Design review of the part built by this model. Coordinates are the model's own, in mm. Face numbers are marked on the shaded views. A direction names the side the tool comes from. Give positions to 0.01 mm unless a question says otherwise; leave off trailing zeros. Write each loop counter-clockwise with the first axis right and the second up, starting at its lowest first coordinate (ties: lowest second). Pieces come first, ordered by that corner, then holes. Notation, with made-up numbers: (-3, -9.75) -> (17, -9.75) arc R15 cw to (17, 0.25) -> close; hole circle Ø7 at (69, -18). An arc over 180 degrees is marked (long way). Use CSV: the item, a comma, the result in double quotes.
```python
from build123d import *

# Parameters (mm, degrees)
EXTRUDE_1_DEPTH     = 30
SKETCH_2_W          = 8
SKETCH_2_H          = 40
EXTRUDE_2_DEPTH     = 100
SKETCH_3_R          = 20
CUT_EXTRUDE_1_DEPTH = 211.428135001
SKETCH_5_W          = 87.00766185
SKETCH_5_H          = 105.192301749
CUT_EXTRUDE_2_DEPTH = 10


with BuildPart() as part:
    # 草图1 → 凸台-拉伸1 (new body)
    with BuildSketch(Plane(origin=(0, 0, 0), x_dir=(1, 0, 0), z_dir=(0, 1, 0))):
        with BuildLine():
            Line((-74, 20), (-71.246052522, 20))
            ThreePointArc((-71.246052522, 20), (0, 74), (71.246052522, 20))
            Line((71.246052522, 20), (74, 20))
            Line((74, 20), (74, -20))
            Line((74, -20), (66, -20))
            Line((66, -20), (66, 0))
            ThreePointArc((66, 0), (0, 66), (-66, 0))
            Line((-66, 0), (-66, -20))
            Line((-66, -20), (-74, -20))
            Line((-74, -20), (-74, 20))
        make_face()
    extrude(amount=EXTRUDE_1_DEPTH)

    # 草图2 → 凸台-拉伸2 (add)
    with BuildSketch(Plane(origin=(0, 30, 0), x_dir=(1, 0, 0), z_dir=(0, 1, 0))):
        with Locations((-70, 0)):
            Rectangle(SKETCH_2_W, SKETCH_2_H)
        with Locations((70, 0)):
            Rectangle(SKETCH_2_W, SKETCH_2_H)
    extrude(amount=EXTRUDE_2_DEPTH)

    # 草图3 → 切除-拉伸1 (cut, through all)
    with BuildSketch(Plane.ZY.offset(74)):
        with Locations((0, 146)):
            Circle(SKETCH_3_R)
    extrude(amount=-CUT_EXTRUDE_1_DEPTH, mode=Mode.SUBTRACT)

    # 草图5 → 切除-拉伸2 (cut)
    with BuildSketch(Plane(origin=(74, 0, 0), x_dir=(0, 0, -1), z_dir=(1, 0, 0))):
        with Locations((-23.503830925, 82.596150874)):
            Rectangle(SKETCH_5_W, SKETCH_5_H)
    extrude(amount=-CUT_EXTRUDE_2_DEPTH, mode=Mode.SUBTRACT)


solid = part.part
```
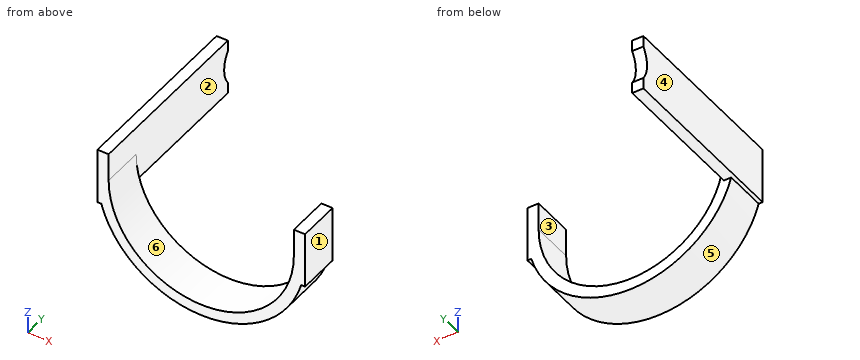
(1) For line 1 along X through (y, z) = (56, -5); line 2 along Z through (x, y) = (-19, 15); line 3 along Z through (x, y) = (-54, 29), list the stretches that pass through material, from the lowest coordinate up. Write a range as [from, to].
Established:
line 1,"x = [-74, -66]"
line 2,"z = [-71.52, -63.21]"
line 3,"z = [-50.6, -37.95]"
(2) Tool access review of the marked faces 1, 2 and 3: name each direction out of +Z, -Z, +X, -X, +Y, -Y from which nothing blocks a thin tool from reaching the whole face with its end or side.
Established:
face 1,"+Z, -Z, +X, +Y, -Y"
face 2,"+Z, +Y"
face 3,"+Z, +Y, -Y"
(3) Mouldability with a two-part tool opening along X and no side actions: class the marked faces 4, 5 and 6 as +X half, -X half, draft (parallel to the pull), parting line (faces both ways), or undercut.
Established:
face 4,"-X half"
face 5,"parting line"
face 6,"undercut"
(4) Take a section at C-C (x = 0). Write out the cut boundary in (y, z).
Established:
outline,"(0, -74) -> (30, -74) -> (30, -66) -> (0, -66) -> close"
(5) Take a section at A-A (z = -37). Write out the cut boundary in (x, y).
Established:
outline,"(-64.09, 0) -> (-54.65, 0) -> (-54.65, 30) -> (-64.09, 30) -> close; (54.65, 0) -> (64.09, 0) -> (64.09, 30) -> (54.65, 30) -> close"
(6) Clearance check with a flat-ended pin moving along its axis: pin 1 (4 mm diameter, centred on x = -70.5, y = 39.5, fed in from -Z). State where the tip first meets the part, or that it passes through.
Established:
pin 1,"stops at z = -20"
(7) Take a section at D-D (z = 10). Write out the cut boundary in (x, y), then the cut area to 3 significant figures.
Established:
outline,"(-74, 0) -> (-66, 0) -> (-66, 128.68) -> (-74, 128.68) -> close; (66, 0) -> (74, 0) -> (74, 30) -> (66, 30) -> close"
area,"1,270 mm2"
(8) Take a section at B-B (y = 12). Write out the cut boundary in (x, z).
Established:
outline,"(-74, -20) -> (-71.25, -20) arc R74 ccw to (71.25, -20) -> (74, -20) -> (74, 20) -> (66, 20) -> (66, 0) arc R66 cw to (-66, 0) -> (-66, 20) -> (-74, 20) -> close"
